from build123d import *

# Parameters (mm, degrees)
SKETCH_W          = 44.5
SKETCH_H          = 44.5
PAD_DEPTH         = 4.7
FILLET_R          = 2
FILLET001_R       = 1
SKETCH001_R       = 0.75
PAD001_DEPTH      = 2
PAD001_DEPTH_BACK = 1
FILLET002_R       = 0.25


with BuildPart() as part:
    # Sketch → Pad (new body)
    with BuildSketch(Plane.XY):
        with Locations((-22.25, 22.25)):
            Rectangle(SKETCH_W, SKETCH_H)
    extrude(amount=PAD_DEPTH)

    # Fillet
    fillet_edges = [part.edges().sort_by_distance(p)[0] for p in [
        (0, 44.5, 2.35),
        (0, 0, 2.35),
        (0, 22.25, 0),
        (0, 22.25, 4.7),
    ]]
    fillet(fillet_edges, radius=FILLET_R)

    # Fillet001
    fillet001_edges = [part.edges().sort_by_distance(p)[0] for p in [
        (-23.25, 44.5, 0),
        (-2, 44.5, 2.35),
        (-44.5, 44.5, 2.35),
        (-23.25, 44.5, 4.7),
        (-44.5, 0, 2.35),
        (-44.5, 22.25, 0),
        (-44.5, 22.25, 4.7),
        (-23.25, 0, 0),
        (-2, 0, 2.35),
        (-23.25, 0, 4.7),
    ]]
    fillet(fillet001_edges, radius=FILLET001_R)

    # Sketch001 (on Face1 of Fillet001) → Pad001 (join, two sides)
    with BuildSketch(Plane(origin=(0, 44.5, 0), x_dir=(-1, 0, 0), z_dir=(0, 1, 0))) as pad001_sk:
        with Locations((0.996389, 2.278105)):
            Circle(SKETCH001_R)
    extrude(amount=PAD001_DEPTH)
    extrude(pad001_sk.sketch, amount=-PAD001_DEPTH_BACK)

    # Fillet002
    fillet002_edges = [part.edges().sort_by_distance(p)[0] for p in [
        (-0.246389, 46.5, 2.278105),
    ]]
    fillet(fillet002_edges, radius=FILLET002_R)


solid = part.part
The listing builds one solid part. Answer for the finished solid, in the listing's coordinates (mm). A direction names the side the tool comes from. Give positions to 0.01 mm unless a question says otherwise; leave off trailing zeros. Loops run counter-clockwise (first coordinate to the right, second up) from the corner with the lowest first, then second, coordinate; pieces in that order, holes last.
Item 1: This flat-tipped pin is pushed along its axis until it touches: pin 1 Ø1.4 at (x, z) = (-31, 1.5) entering from +Y. Where does it stop, or does it pass through?
Derived:
pin 1: stops at y = 44.5
Item 2: A tool of negligible diameter and unlimited length cuts with its end or side. For faces 1 (the flat face through (-23, 44.5, 2)), 2 (the flat face through (-44.5, 22, 2)), 3 (the cylindrical face through (-0.247, 45.2, 2.311)), from which of +Z, -Z, +X, -X, +Y, -Y can it reach the whole face along a straight path? Write none if from no direction.
Derived:
face 1: +Z, -Z, -X, +Y
face 2: +Z, -Z, -X, +Y, -Y
face 3: +Y
Item 3: A cutting plane is placed at A-A (x = -37). Give the vertices of the cut face in (y, z).
Derived:
outline: (0, 1) arc R1 ccw to (1, 0) - (43.5, 0) arc R1 ccw to (44.5, 1) - (44.5, 3.7) arc R1 ccw to (43.5, 4.7) - (1, 4.7) arc R1 ccw to (0, 3.7) - close
Item 4: Find the intervals of material crossed by line 1 along Y through (x, z) = (-22, 2.5); line 2 along X through (y, z) = (43.5, 1.85); line 3 along X through (y, z) = (15, 3), in increasing order.
Derived:
line 1: y = 0 to 44.5
line 2: x = -44.5 to -0.27
line 3: x = -44.5 to -0.02
